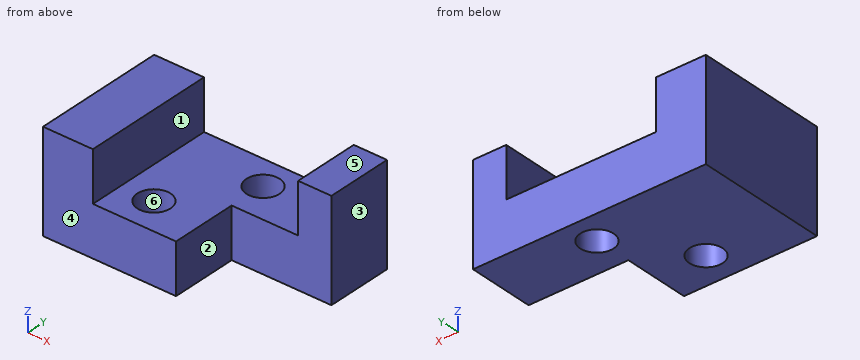
```python
from build123d import *

# Parameters (mm, degrees)
F1_DEPTH = 50.8
F2_W     = 38.1
F2_H     = 25.4
F3_DEPTH = 39.21464
F5_D     = 12.7
F7_D     = 12.7


with BuildPart() as f1:
    # F0 (on Front) → F1 (new body)
    with BuildSketch(Plane.XZ):
        Polygon((-80.216871, 9.032293), (-99.266871, 9.032293), (-99.266871, -29.067707), (-10.366871, -29.067707), (-10.366871, 9.032293), (-23.066871, 9.032293), (-23.066871, -10.017707), (-80.216871, -10.017707), align=None)
    extrude(amount=-F1_DEPTH)

    # F2 (on face) → F3 (cut)
    with BuildSketch(Plane(origin=(0, 0, -29.067707), x_dir=(1, 0, 0), z_dir=(0, 0, -1))):
        with Locations((-29.416871, -12.7)):
            Rectangle(F2_W, F2_H)
    extrude(amount=-F3_DEPTH, mode=Mode.SUBTRACT)

    # F5 (through all)
    with Locations(Plane.XY.offset(-10.017707)):
        with Locations((-67.516871, 12.7)):
            Hole(F5_D / 2)

    # F7 (through all)
    with Locations(Plane.XY.offset(-10.017707)):
        with Locations((-48.063979, 39.275229)):
            Hole(F7_D / 2)


solid = f1.part
```
Check sheet for the modelled part. Datum: model origin and axes. Units: mm. Face numbers are marked on the shaded views. A direction names the side the tool comes from. Give positions to 0.01 mm unless a question says otherwise; leave off trailing zeros. Loops run counter-clockwise (first coordinate to the right, second up) from the corner with the lowest first, then second, coordinate; pieces in that order, holes last. Notation, with made-up numbers: M -34.75,85 L 11.25,85 A27 cw 11.25,108 Z; hole C -25,-25.5 d5. An arc over 180 degrees is marked long. Answer as CSV lines item,"result".
Item 1: Sectioned sample at D-D, the plane x = -35.5. Enter the section's corners in (y, z), then the cut area to 3 significant figures.
Reply:
outline,"M 25.4,-29.07 L 50.8,-29.07 L 50.8,-10.02 L 25.4,-10.02 Z"
area,"484 mm^2"
Item 2: Depth check by flat-ended pin: pin 1 Ø12 at (x, z) = (-23.5, -16) entering from -Y; pin 2 Ø5.5 at (y, z) = (10.5, -16.5) entering from +X; pin 3 Ø14.5 at (x, y) = (-48.06, 39.28) entering from +Z. Enter the tip coordinate at first touch or a pass-through.
Reply:
pin 1,"y = 25.4"
pin 2,"x = -48.47"
pin 3,"z = -10.02"
Item 3: Sectioned sample at C-C, the plane y = 27. Enter the section's corners in (x, z), then the cut area to 3 significant figures.
Reply:
outline,"M -99.27,-29.07 L -10.37,-29.07 L -10.37,9.03 L -23.07,9.03 L -23.07,-10.02 L -80.22,-10.02 L -80.22,9.03 L -99.27,9.03 Z"
area,"2,300 mm^2"
Item 4: Sectioned sample at A-A, the plane y = 12.7. Enter the section's corners in (x, z).
Reply:
outline,"M -99.27,-29.07 L -73.87,-29.07 L -73.87,-10.02 L -80.22,-10.02 L -80.22,9.03 L -99.27,9.03 Z; M -61.17,-29.07 L -48.47,-29.07 L -48.47,-10.02 L -61.17,-10.02 Z"
Item 5: Scan lines: L1, parallel to Y at x = -19, z = -5.5; L2, parallel to Z at x = -74.5, y = 9; L3, parallel to X at y = 15, z = -8. Record each from-to range of solid material in increasing order.
Reply:
L1,"25.4 to 50.8"
L2,"-29.07 to -10.02"
L3,"-99.27 to -80.22"
Item 6: Set-up check for the marked faces 1, 2 and 3: record each of +Z, -Z, +X, -X, +Y, -Y from which the full face is reachable in a straight line by a thin tool's end or side.
Reply:
face 1,"+Z, +Y, -Y"
face 2,"+Z, -Z, +X, -Y"
face 3,"+Z, -Z, +X, +Y, -Y"
Item 7: Sectioned sample at B-B, the plane z = -3.5. Enter the section's corners in (x, y), then the cut area to 3 significant figures.
Reply:
outline,"M -99.27,0 L -80.22,0 L -80.22,50.8 L -99.27,50.8 Z; M -23.07,25.4 L -10.37,25.4 L -10.37,50.8 L -23.07,50.8 Z"
area,"1,290 mm^2"
Item 8: Draft check along Y on the marked faces 4, 5 and 6. Enter one of: pulls with the +Y half, pulls with the -Y half, needs draft (parallel to the pull), parting line crosses it, or undercut.
Reply:
face 4,"pulls with the -Y half"
face 5,"needs draft"
face 6,"undercut"
